```python
from build123d import *

# Parameters (mm, degrees)
BOSS_EXTRUDE1_DEPTH      = 42.5
BOSS_EXTRUDE1_DEPTH_BACK = 15
SKETCH1_W                = 40
SKETCH1_H                = 65
SKETCH3_W                = 22.5
SKETCH3_H                = 50
CUT_EXTRUDE2_DEPTH       = 30
SKETCH4_R                = 4.5
CUT_EXTRUDE3_DEPTH       = 10
SKETCH5_W                = 35
SKETCH5_H                = 25
BOSS_EXTRUDE3_DEPTH      = 15
SKETCH6_R                = 3
CUT_EXTRUDE4_DEPTH       = 15
CUT_EXTRUDE5_DEPTH       = 108.964114408
BOSS_EXTRUDE4_DEPTH      = 10
BOSS_EXTRUDE5_OUTLINE_R  = 3
BOSS_EXTRUDE5_DEPTH      = 50
BOSS_EXTRUDE6_START      = -50
SKETCH11_R               = 3
BOSS_EXTRUDE6_DEPTH      = 50
SKETCH12_W               = 14
SKETCH12_H               = 65
SKETCH12_R               = 3.1
SKETCH12_W_2             = 75
SKETCH12_H_2             = 14
BOSS_EXTRUDE7_DEPTH      = 5
SKETCH13_R               = 1.6
CUT_EXTRUDE6_DEPTH       = 115.988042857
CUT_EXTRUDE7_DEPTH       = 11.5
CUT_EXTRUDE7_DEPTH_BACK  = 11.5
SKETCH14_W               = 43.75
SKETCH14_H               = 50
CUT_EXTRUDE8_DEPTH       = 30
CUT_EXTRUDE9_DEPTH       = 115.988042857
CUT_EXTRUDE10_DEPTH      = 18
SKETCH18_W               = 31
SKETCH18_H               = 12
SKETCH18_R               = 2.1
BOSS_EXTRUDE8_DEPTH      = 5
FILLET2_R                = 1
SKETCH19_W               = 9.25
SKETCH19_H               = 10
CUT_EXTRUDE11_DEPTH      = 10
CHAMFER1_SIZE            = 1
CHAMFER2_SIZE            = 1


# Read off the part's stored shape, not the designer's step: Boss-Extrude5
# Some blends are built 0.0001 mm under size
with BuildPart() as part:
    # Sketch1 → Boss-Extrude1 (new, two sides: drawn at the far end of the back side and taken through both)
    with BuildSketch(Plane.XY.offset(-BOSS_EXTRUDE1_DEPTH_BACK)):
        with Locations((20, 32.5)):
            Rectangle(SKETCH1_W, SKETCH1_H)
    extrude(amount=BOSS_EXTRUDE1_DEPTH + BOSS_EXTRUDE1_DEPTH_BACK)

    # Sketch3 → Cut-Extrude2 (cut)
    with BuildSketch(Plane(origin=(40, 0, 0), x_dir=(0, 0, -1), z_dir=(1, 0, 0))):
        with Locations((-11.25, 40)):
            Rectangle(SKETCH3_W, SKETCH3_H)
    extrude(amount=-CUT_EXTRUDE2_DEPTH, mode=Mode.SUBTRACT)

    # Sketch4 → Cut-Extrude3 (cut)
    with BuildSketch(Plane(origin=(10, 0, 0), x_dir=(0, 0, -1), z_dir=(1, 0, 0))):
        with Locations((-11.25, 26.5)):
            Circle(SKETCH4_R)
    extrude(amount=-CUT_EXTRUDE3_DEPTH, mode=Mode.SUBTRACT)

    # Sketch5 → Boss-Extrude3 (add)
    with BuildSketch(Plane.XZ):
        with Locations((57.5, 30)):
            Rectangle(SKETCH5_W, SKETCH5_H)
    extrude(amount=-BOSS_EXTRUDE3_DEPTH)

    # Sketch6 → Cut-Extrude4 (cut)
    with BuildSketch(Plane.XZ):
        with Locations(Location((32, 29.5, 0), (0, 0, 270))):
            Circle(SKETCH6_R)
        with Locations(Location((64, 29.5, 0), (0, 0, 270))):
            Circle(SKETCH6_R)
    extrude(amount=-CUT_EXTRUDE4_DEPTH, mode=Mode.SUBTRACT)

    # Sketch8 → Cut-Extrude5 (cut, through all)
    with BuildSketch(Plane.XZ):
        Polygon((48.25, 17.5), (42.75, 17.5), (42.75, 23), (53.75, 23), (53.75, 17.5), align=None)
    extrude(amount=-CUT_EXTRUDE5_DEPTH, mode=Mode.SUBTRACT)

    # Sketch9 → Boss-Extrude4 (add)
    with BuildSketch(Plane.XY.offset(42.5)):
        Polygon((0, 65), (0, 0), (75, 0), (75, 15), (40, 15), (40, 65), align=None)
    extrude(amount=BOSS_EXTRUDE4_DEPTH)

    # Boss-Extrude5 outline → Boss-Extrude5 (add)
    with BuildSketch(Plane(origin=(0, 15, 0), x_dir=(1, 0, 0), z_dir=(0, 1, 0))):
        Polygon((75, -52.5), (75, -22.5), (53.75, -22.5), (53.75, -23), (42.75, -23), (42.75, -22.5), (40, -22.5), (40, -52.5), align=None)
        with Locations((64, -29.5)):
            Circle(BOSS_EXTRUDE5_OUTLINE_R, mode=Mode.SUBTRACT)
    extrude(amount=BOSS_EXTRUDE5_DEPTH)

    # Sketch11 → Boss-Extrude6 (add)
    with BuildSketch(Plane(origin=(0, 65, 0), x_dir=(1, 0, 0), z_dir=(0, 1, 0)).offset(BOSS_EXTRUDE6_START)):
        with Locations(Location((64, -29.5, 0), (0, 0, 90))):
            Circle(SKETCH11_R)
    extrude(amount=BOSS_EXTRUDE6_DEPTH)

    # Sketch12 → Boss-Extrude7 (add)
    # profile 1 of 2: a face of its own
    with BuildSketch(Plane.XY.offset(52.5)):
        with Locations((82, 32.5)):
            Rectangle(SKETCH12_W, SKETCH12_H)
        with Locations((82, 53)):
            Circle(SKETCH12_R, mode=Mode.SUBTRACT)
        with Locations((82, 12)):
            Circle(SKETCH12_R, mode=Mode.SUBTRACT)
    # profile 2 of 2: a face of its own
    with BuildSketch(Plane.XY.offset(52.5)):
        with Locations((37.5, -7)):
            Rectangle(SKETCH12_W_2, SKETCH12_H_2)
        with Locations((12, -7)):
            Circle(SKETCH12_R, mode=Mode.SUBTRACT)
        with Locations((63, -7)):
            Circle(SKETCH12_R, mode=Mode.SUBTRACT)
    extrude(amount=-BOSS_EXTRUDE7_DEPTH)

    # Sketch13 → Cut-Extrude6 (cut, through all)
    with BuildSketch(Plane(origin=(10, 0, 0), x_dir=(0, 0, -1), z_dir=(1, 0, 0))):
        with Locations((-2.5, 47)):
            Circle(SKETCH13_R)
        with Locations((-20, 47)):
            Circle(SKETCH13_R)
    extrude(amount=-CUT_EXTRUDE6_DEPTH, mode=Mode.SUBTRACT)

    # Sketch14 → Cut-Extrude7 (cut, two sides: drawn at the far end of the back side and taken through both)
    with BuildSketch(Plane(origin=(0, 0, 11.25), x_dir=(-1, 0, 0), z_dir=(0, 0, -1)).offset(-CUT_EXTRUDE7_DEPTH_BACK)):
        with Locations((-31.875, 40)):
            Rectangle(SKETCH14_W, SKETCH14_H)
    extrude(amount=CUT_EXTRUDE7_DEPTH + CUT_EXTRUDE7_DEPTH_BACK, mode=Mode.SUBTRACT)

    # Sketch15 → Cut-Extrude8 (cut)
    with BuildSketch(Plane(origin=(40, 0, 0), x_dir=(0, 0, -1), z_dir=(1, 0, 0))):
        Polygon((-11.25, 15), (-8.25, 15), (-8.25, 9), (-14.25, 9), (-14.25, 15), align=None)
    extrude(amount=-CUT_EXTRUDE8_DEPTH, mode=Mode.SUBTRACT)

    # Sketch16 → Cut-Extrude9 (cut, through all)
    with BuildSketch(Plane(origin=(10, 0, 0), x_dir=(0, 0, -1), z_dir=(1, 0, 0))):
        Polygon((-11.25, 65), (-8.25, 65), (-8.25, 50), (-14.25, 50), (-14.25, 65), align=None)
    extrude(amount=-CUT_EXTRUDE9_DEPTH, mode=Mode.SUBTRACT)

    # Sketch17 → Cut-Extrude10 (cut)
    with BuildSketch(Plane.ZY):
        with BuildLine():
            Line((28.25, 26.5), (28.25, 0))
            Line((28.25, 0), (-5.75, 0))
            Line((-5.75, 0), (-5.75, 26.5))
            ThreePointArc((-5.75, 26.5), (11.25, 43.5), (28.25, 26.5))
        make_face()
    extrude(amount=-CUT_EXTRUDE10_DEPTH, mode=Mode.SUBTRACT)

    # Sketch18 → Boss-Extrude8 (add)
    # profile 1 of 3: a face of its own
    with BuildSketch(Plane(origin=(78.326188017, 6.6, -27.619079409), x_dir=(-1, 0, 0), z_dir=(0, -1, 0))):
        Polygon((60.326188017, -28.604062705), (60.326188017, -33.604062705), (65.326188017, -33.604062705), align=None)
    # profile 2 of 3: a face of its own
    with BuildSketch(Plane(origin=(78.326188017, 6.6, -27.619079409), x_dir=(-1, 0, 0), z_dir=(0, -1, 0))):
        Polygon((65.326188017, -45.604062705), (60.326188017, -45.604062705), (60.326188017, -50.604062705), align=None)
    # profile 3 of 3: a face of its own
    with BuildSketch(Plane(origin=(78.326188017, 6.6, -27.619079409), x_dir=(-1, 0, 0), z_dir=(0, -1, 0))):
        with Locations((75.826188017, -39.604062705)):
            Rectangle(SKETCH18_W, SKETCH18_H)
        with Locations(Location((85.648688017, -38.869079409, 0), (0, 0, 90))):
            Circle(SKETCH18_R, mode=Mode.SUBTRACT)
        with Locations(Location((65.828688017, -38.869079409, 0), (0, 0, 90))):
            Circle(SKETCH18_R, mode=Mode.SUBTRACT)
    extrude(amount=BOSS_EXTRUDE8_DEPTH)

    # Fillet2
    fillet2_edges = [part.edges().sort_by_distance(p)[0] for p in [
        (0, 43.5, 11.25),
        (0, 13.25, -5.75),
        (0, 13.25, 28.25),
    ]]
    fillet(fillet2_edges, radius=FILLET2_R)

    # Sketch19 → Cut-Extrude11 (cut)
    with BuildSketch(Plane.ZY):
        with Locations((-10.375, 5)):
            Rectangle(SKETCH19_W, SKETCH19_H)
    extrude(amount=-CUT_EXTRUDE11_DEPTH, mode=Mode.SUBTRACT)

    # Chamfer1
    # the kernel refuses this chamfer: 1 mm, written as the material it adds along each edge
    with BuildSketch(Plane(origin=(75, 0, 47.5), x_dir=(-0.027495876610582105, 0, -0.999621916911297), z_dir=(0, 1, 0))) as chamfer1_piece_1:
        Polygon((CHAMFER1_SIZE * 0.999621916911, -CHAMFER1_SIZE * 0.0274958766106), (-CHAMFER1_SIZE * 0.0274958766106, -CHAMFER1_SIZE * 0.999621916911), (0, 0), align=None)
    extrude(amount=65)

    # Chamfer2
    chamfer2_edges = [part.edges().sort_by_distance(p)[0] for p in [
        (37.5, 0, 47.5),
    ]]
    chamfer(chamfer2_edges, length=CHAMFER2_SIZE - 0.0001)  # a hair under: the kernel refuses the full size

    # Chamfer3
    # the kernel refuses this chamfer: 1 mm, written as the material it adds along each edge
    with BuildSketch(Plane(origin=(75, 0, 52.5), x_dir=(0.9996219169112968, 0.02749587661058591, 0), z_dir=(0, 0, -1))) as chamfer3_piece_1_section:
        with BuildLine():
            Line((1.028673195, 0), (-0.056547155, 1.027117794))
            Line((-0.056547155, 1.027117794), (-0.076539593, 1.026567876))
            ThreePointArc((-0.076539593, 1.026567876), (-0.034129227, 0.51339783), (-0.019992438, -0.000549918))
            Line((-0.019992438, -0.000549918), (0.000549918, -0.019992438))
            ThreePointArc((0.000549918, -0.019992438), (0.514497665, -0.00585565), (1.029223113, -0.019992438))
            Line((1.029223113, -0.019992438), (1.028673195, 0))
        make_face()
    chamfer3_piece_1 = extrude(amount=8.571582988, mode=Mode.PRIVATE)
    chamfer3_piece_1 = split(chamfer3_piece_1, bisect_by=Plane(origin=(75.329792283, -0.329792248, 47.5), z_dir=(0, 0, 1)), keep=Keep.TOP, mode=Mode.PRIVATE)
    add(chamfer3_piece_1)
    with BuildSketch(Plane(origin=(75, 0, 52.5), x_dir=(0.9996219169112968, 0.02749587661058591, 0), z_dir=(0, 0, -1))) as chamfer3_piece_2_section:
        with BuildLine():
            Line((1.028673195, 0), (-0.056547155, 1.027117794))
            Line((-0.056547155, 1.027117794), (-0.076539593, 1.026567876))
            ThreePointArc((-0.076539593, 1.026567876), (-0.034129227, 0.51339783), (-0.019992438, -0.000549918))
            Line((-0.019992438, -0.000549918), (0.000549918, -0.019992438))
            ThreePointArc((0.000549918, -0.019992438), (0.514497665, -0.00585565), (1.029223113, -0.019992438))
            Line((1.029223113, -0.019992438), (1.028673195, 0))
        make_face()
    chamfer3_piece_2 = extrude(amount=8.571582988, mode=Mode.PRIVATE)
    chamfer3_piece_2 = split(chamfer3_piece_2, bisect_by=Plane(origin=(74.967608751, -1.017389606, 47.5), z_dir=(0, 0, 1)), keep=Keep.TOP, mode=Mode.PRIVATE)
    chamfer3_piece_2 = split(chamfer3_piece_2, bisect_by=Plane(origin=(74.967608751, -1.013017205, 47.513117205), z_dir=(0, -0.7071067811865464, -0.7071067811865488)), keep=Keep.TOP, mode=Mode.PRIVATE)
    add(chamfer3_piece_2)
    with BuildSketch(Plane(origin=(75, 0, 52.5), x_dir=(0.9996219169112968, 0.02749587661058591, 0), z_dir=(0, 0, -1))) as chamfer3_piece_3_section:
        with BuildLine():
            Line((1.028673195, 0), (-0.056547155, 1.027117794))
            Line((-0.056547155, 1.027117794), (-0.076539593, 1.026567876))
            ThreePointArc((-0.076539593, 1.026567876), (-0.034129227, 0.51339783), (-0.019992438, -0.000549918))
            Line((-0.019992438, -0.000549918), (0.000549918, -0.019992438))
            ThreePointArc((0.000549918, -0.019992438), (0.514497665, -0.00585565), (1.029223113, -0.019992438))
            Line((1.029223113, -0.019992438), (1.028673195, 0))
        make_face()
    chamfer3_piece_3 = extrude(amount=8.571582988, mode=Mode.PRIVATE)
    chamfer3_piece_3 = split(chamfer3_piece_3, bisect_by=Plane(origin=(75.495112372, -0.283467256, 46.995112372), z_dir=(-0.7071067811862649, 0, 0.7071067811868302)), keep=Keep.TOP, mode=Mode.PRIVATE)
    chamfer3_piece_3 = split(chamfer3_piece_3, bisect_by=Plane(origin=(75.283503511, -0.283467256, 47.5), z_dir=(0, 0, -1)), keep=Keep.TOP, mode=Mode.PRIVATE)
    chamfer3_piece_3 = split(chamfer3_piece_3, bisect_by=Plane(origin=(75.283503511, -0.495044244, 46.995144244), z_dir=(0, 0.7071067811865464, 0.7071067811865488)), keep=Keep.TOP, mode=Mode.PRIVATE)
    add(chamfer3_piece_3)
    with BuildSketch(Plane(origin=(75, 0, 52.5), x_dir=(0.9996219169112968, 0.02749587661058591, 0), z_dir=(0, 0, -1))) as chamfer3_piece_4_section:
        with BuildLine():
            Line((1.028673195, 0), (-0.056547155, 1.027117794))
            Line((-0.056547155, 1.027117794), (-0.076539593, 1.026567876))
            ThreePointArc((-0.076539593, 1.026567876), (-0.034129227, 0.51339783), (-0.019992438, -0.000549918))
            Line((-0.019992438, -0.000549918), (0.000549918, -0.019992438))
            ThreePointArc((0.000549918, -0.019992438), (0.514497665, -0.00585565), (1.029223113, -0.019992438))
            Line((1.029223113, -0.019992438), (1.028673195, 0))
        make_face()
    chamfer3_piece_4 = extrude(amount=8.571582988, mode=Mode.PRIVATE)
    chamfer3_piece_4 = split(chamfer3_piece_4, bisect_by=Plane(origin=(76.01307363, 0.032413897, 47.51307363), z_dir=(0.7071067811862649, 0, -0.7071067811868302)), keep=Keep.TOP, mode=Mode.PRIVATE)
    chamfer3_piece_4 = split(chamfer3_piece_4, bisect_by=Plane(origin=(76.017431506, 0.032413897, 47.5), z_dir=(0, 0, 1)), keep=Keep.TOP, mode=Mode.PRIVATE)
    add(chamfer3_piece_4)


solid = part.part
```
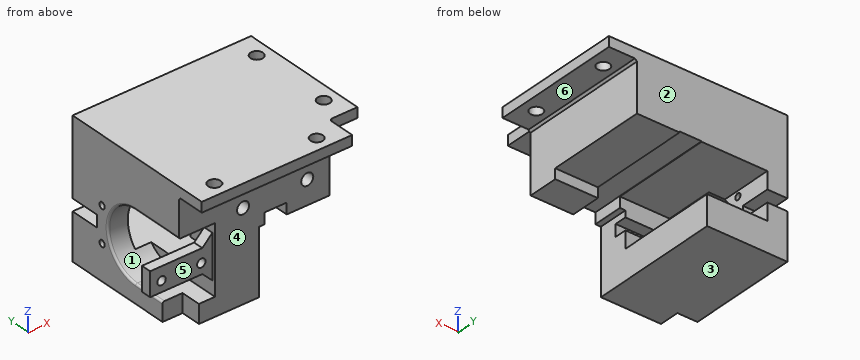
Here's how the part is built. I have some questions about the finished solid (model axes, mm). Face numbers are marked on the shaded views. A direction names the side the tool comes from. Coordinates: 2 decimals unless noted, no trailing zeros. Order: outer loops, then holes, each group sorted by start corner. A loop starts at its lowest first (then second) coordinate and runs counter-clockwise, first axis right, second up.
1) I need wall thicknesses on line 1 (X direction, y = 3.8, z = 11.25); line 2 (Y direction, x = 63, z = 49); line 3 (Z direction, x = 19.5, y = 54). Which ranges of each line are inside material? Lowest first, please.
2) We'd pull the mould along Z, two halves only. Please class the marked faces 1, 2 and 3: +Z half, -Z half, draft (parallel to the pull), parting line (faces both ways), or undercut.
3) Imagine slicing it at C-C on y = 23.5. List the corners of the cut face in (x, z) for me.
4) Will these pins go through, and if not, where does the flat tip stop? pin 1 (12 mm diameter, centred on x = 64, y = 8, fed in from -Z); pin 2 (5 mm diameter, centred on y = 48.5, z = 10, fed in from +X); pin 3 (9.5 mm diameter, centred on x = 32, z = 29.5, fed in from -Y).
5) Imagine slicing it at A-A on y = -7. List the corners of the cut face in (x, z) for me, and give its area (3 significant figures).
6) Imagine slicing it at D-D on z = -8.5. List the corners of the cut face in (x, y) for me, and give its area (3 significant figures).
7) Imagine slicing it at B-B on x = 64. List the corners of the cut face in (y, z) for me.
8) Which directions (+Z, -Z, +X, -X, +Y, -Y) give clear straight access to the entire face, cutting with the end or side of a thin tool? Please do the marked faces 4, 5 and 6.
Response values:
1. line 1: x = -13 to -9.42, -5.22 to 10.4, 14.6 to 40
1. line 2: y = -14 to -10.1, -3.9 to 65
1. line 3: z = -15 to -0.25, 22.75 to 52.5
2. face 1: undercut
2. face 2: draft
2. face 3: -Z half
3. outline: (0, -15) - (40, -15) - (40, -0.25) - (18, -0.25) - (18, -5.75) - (1, -5.75) arc R1 ccw to (0, -6.75) - close; (0, 29.25) arc R1 ccw to (1, 28.25) - (18, 28.25) - (18, 22.75) - (42.75, 22.75) - (42.75, 23) - (53.75, 23) - (53.75, 22.5) - (75, 22.5) - (75, 46.5) - (76, 47.5) - (89, 47.5) - (89, 52.5) - (0, 52.5) - close
4. pin 1: stops at z = 17.5
4. pin 2: stops at x = 10
4. pin 3: stops at y = 0
5. outline: (0, 47.5) - (8.9, 47.5) - (8.9, 52.5) - (0, 52.5) - close; (15.1, 47.5) - (59.9, 47.5) - (59.9, 52.5) - (15.1, 52.5) - close; (66.1, 47.5) - (75, 47.5) - (75, 52.5) - (66.1, 52.5) - close
5. area: 313 mm2
6. outline: (0, 10) - (10, 10) - (10, 0) - (40, 0) - (40, 65) - (0, 65) - close
6. area: 2,500 mm2
7. outline: (-14, 47.5) - (-9.93, 47.5) - (-9.93, 52.5) - (-14, 52.5) - close; (-4.07, 47.5) - (-1, 47.5) - (0, 46.5) - (0, 32.5) - (15, 32.5) - (15, 26.5) - (0, 26.5) - (0, 17.5) - (15, 17.5) - (15, 22.5) - (65, 22.5) - (65, 52.5) - (-4.07, 52.5) - close
8. face 4: -Z, +X, -X, -Y
8. face 5: -X, -Y
8. face 6: -Z, +X, +Y, -Y
